Work out the finished part from the listing and answer in its coordinate system (mm). Coordinates: 2 decimals unless noted, no trailing zeros. Order: outer loops, then holes, each group sorted by start corner. A loop starts at its lowest first (then second) coordinate and runs counter-clockwise, first axis right, second up. Notation, with made-up numbers: M 89.5,-36.75 L 101.5,-36.75 A19 cw 101.5,-11.75 Z; hole C -12.75,-20 d9. An arc over 180 degrees is marked long. Use a Markdown table: item, result.
from build123d import *

# Parameters (mm, degrees)
SKETCH1_R           = 2.5
BOSS_EXTRUDE1_DEPTH = 11
SKETCH2_R           = 0.25
BOSS_EXTRUDE2_DEPTH = 5
SKETCH3_R           = 1.5
FILLET1_R           = 1
FILLET2_R           = 0.5
FILLET3_R           = 0.5


with BuildPart() as part:
    # Sketch1 → Boss-Extrude1 (new body)
    with BuildSketch(Plane(origin=(0, 0, 0), x_dir=(1, 0, 0), z_dir=(0, 1, 0))):
        Circle(SKETCH1_R)
    extrude(amount=BOSS_EXTRUDE1_DEPTH)

    # Sketch2 → Boss-Extrude2 (add)
    with BuildSketch(Plane.XZ):
        with Locations((1, 0)):
            Circle(SKETCH2_R)
        with Locations((-1, 0)):
            Circle(SKETCH2_R)
    extrude(amount=BOSS_EXTRUDE2_DEPTH)

    # Sketch3 → Cut-Revolve1 (revolve, cut)
    with BuildSketch(Plane(origin=(0, 0, 0), x_dir=(0, 0, -1), z_dir=(1, 0, 0))):
        with Locations((3.8, 2)):
            Circle(SKETCH3_R)
    revolve(axis=Axis((0, 21.78154861, 0), (0, -1, 0)), mode=Mode.SUBTRACT)

    # Fillet1
    fillet1_edges = [part.edges().sort_by_distance(p)[0] for p in [
        (-1.767766953, 2.748331477, 1.767766953),
        (-1.767766953, 1.251668523, 1.767766953),
    ]]
    fillet(fillet1_edges, radius=FILLET1_R)

    # Fillet2
    fillet2_edges = [part.edges().sort_by_distance(p)[0] for p in [
        (-2.5, 11, 0),
    ]]
    fillet(fillet2_edges, radius=FILLET2_R)

    # Fillet3
    fillet3_edges = [part.edges().sort_by_distance(p)[0] for p in [
        (-2.5, 0, 0),
    ]]
    fillet(fillet3_edges, radius=FILLET3_R)


solid = part.part
1. Section C-C on y = 1.75 is taken. Determine the outline of the cut face in (x, z).
Answers below:
| item | result |
|---|---|
| outline | C 0,0 d4.64 |
2. Section A-A on y = -1.25 is taken. Determine the outline of the cut face in (x, z), then the cut area to 3 significant figures.
Answers below:
| item | result |
|---|---|
| outline | C -1,0 d0.5; C 1,0 d0.5 |
| area | 0.393 mm² |
3. Find the intervals of material crossed by probe 1 along Z at (x, y) = (1.5, 8.75); probe 2 along Y at (x, z) = (0.25, 0.7), in increasing order.
Answers below:
| item | result |
|---|---|
| probe 1 | -2 to 2 |
| probe 2 | 0 to 11 |
4. Section B-B on y = 6.75 is taken. Determine the outline of the cut face in (x, z), then the cut area to 3 significant figures.
Answers below:
| item | result |
|---|---|
| outline | C 0,0 d5 |
| area | 19.6 mm² |
